Geometry: final body of the model. Coordinates: model frame, mm. A direction names the side the tool comes from. Give positions to 0.01 mm unless a question says otherwise; leave off trailing zeros. Order: outer loops, then holes, each group sorted by start corner. A loop starts at its lowest first (then second) coordinate and runs counter-clockwise, first axis right, second up. Notation, with made-up numbers: (24, 64.25) - (59, 64.25) arc R33 ccw to (59, 93.25) - close; hole circle Ø5 at (40.5, -36). An arc over 180 degrees is marked (long way). Put each result on its own line as item: value. Start each with the question number.
1. Ray query, line 1 along Y through (x, z) = (0, 3.75); line 2 along Y through (x, z) = (-3.5, 9); line 3 along X through (y, z) = (5.5, 2). Return the intervals inside material, ascending. Write a range as from..to.
2. Section D-D on x = 8. Return the cut outline in (y, z).
3. Set-up query: faces 1 (the flat face through (2, -5, 0)), 2 (the cylindrical face through (-1.38, -6.2, 5.18)). Return all of +Z, -Z, +X, -X, +Y, -Y with unobstructed straight access to the full face (end or side cutting, diameter ignored); none if empty.
4. Section C-C on z = 1.5. Return the cut outline in (x, y).
5. Section A-A on y = 0. Return the cut outline in (x, z), plus the area to 3 significant figures.
6. First-contact query: P1, Ø2, axis at y = -8.5, z = 5.5, coming from the -X side; P2, Ø1, axis at x = 3, z = 6.5, coming from the +Y side; P3, Ø1.5, axis at x = 1, z = 4, coming from the -Y side. Flat tips, straight axial feed; report the tip coordinate or a pass-through.
7. Mould query, pull axis X, two halves, no side actions, for faces 3 (the cylindrical face through (5.19, -9.98, 4.93)), 4 (the flat face through (2, -6.4, 0.5)), 5 (the flat face through (0, 10, 10)). Classes: pulls with the +X half, pulls with the -X half, needs draft (parallel to the pull), parting line crosses it, or undercut.
from build123d import *

# Parameters (mm, degrees)
F0_R     = 11.25
F0_R_2   = 9.75
F1_DEPTH = 10
F0_R_3   = 6.35
F0_R_4   = 4.8500001431
F2_DEPTH = 0.5


with BuildPart() as f1:
    # F0 (on Top) → F1 (new body)
    with BuildSketch(Plane.XY):
        Circle(F0_R)
        Circle(F0_R_2, mode=Mode.SUBTRACT)
    extrude(amount=F1_DEPTH)



with BuildPart() as f1b:
    # F0 (on Top) → F1, piece 2 (new body)
    with BuildSketch(Plane.XY):
        Circle(F0_R_3)
        Circle(F0_R_4, mode=Mode.SUBTRACT)
    extrude(amount=F1_DEPTH)


with BuildPart() as f1_1:
    add(f1.part)

    add(f1b.part)  # F2 merges F1b
    # F0 (on Top) → F2 (join)
    with BuildSketch(Plane.XY):
        Circle(F0_R_2)
        Circle(F0_R_3, mode=Mode.SUBTRACT)
    extrude(amount=F2_DEPTH)


solid = f1_1.part
Resolved:
1. line 1: -11.25..-9.75, -6.35..-4.85, 4.85..6.35, 9.75..11.25
1. line 2: -10.69..-9.1, -5.3..-3.36, 3.36..5.3, 9.1..10.69
1. line 3: -9.81..-8.05, -3.17..3.17, 8.05..9.81
2. outline: (-7.91, 0) - (7.91, 0) - (7.91, 10) - (5.57, 10) - (5.57, 0.5) - (-5.57, 0.5) - (-5.57, 10) - (-7.91, 10) - close
3. face 1: -Z, +X, -X, +Y, -Y
3. face 2: +Z
4. outline: circle Ø22.5 at (0, 0); circle Ø12.7 at (0, 0); hole circle Ø19.5 at (0, 0); hole circle Ø9.7 at (0, 0)
5. outline: (-11.25, 0) - (-4.85, 0) - (-4.85, 10) - (-6.35, 10) - (-6.35, 0.5) - (-9.75, 0.5) - (-9.75, 10) - (-11.25, 10) - close; (4.85, 0) - (11.25, 0) - (11.25, 10) - (9.75, 10) - (9.75, 0.5) - (6.35, 0.5) - (6.35, 10) - (4.85, 10) - close
5. area: 63.4 mm^2
6. P1: x = -8.39
6. P2: y = 10.97
6. P3: y = -11.25
7. face 3: parting line crosses it
7. face 4: undercut
7. face 5: needs draft
